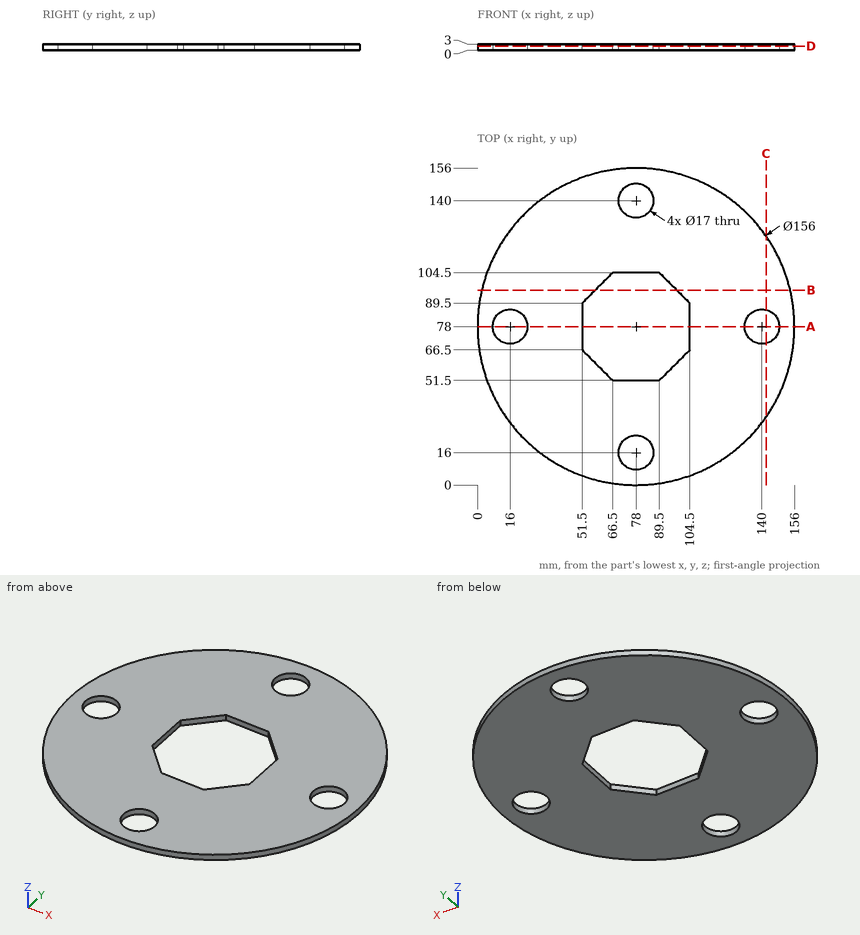
Design review of the part shown in the three views and the two pictorial views. Dimensions are in mm from the part's minimum x, y and z. Give positions to 0.01 mm unless a question says otherwise; leave off trailing zeros. Loops run counter-clockwise (first coordinate to the right, second up) from the corner with the lowest first, then second, coordinate; pieces in that order, holes last. Notation, with made-up numbers: M -2.5,27.5 L 30.5,27.5 A20 cw 30.5,65.5 Z; hole C -14.75,-35 d5. An arc over 180 degrees is marked long. Put each result on its own line as item: value. Start each with the question number.
(1) For pin 1 (0.9 mm diameter, centred on y = 81.5, z = 1.5, fed in from -X); pin 2 (1.5 mm diameter, centred on y = 72.5, z = 1, fed in from +X), all flat-tipped, find the tip position at first contact; note any pin that passes through.
(2) Wall thickness on L1, parallel to Y at x = 78, z = 1.3; L2, parallel to X at y = 79, z = 0.35; L3, parallel to Y at x = 74.5, z = 1.15: over which ranges is each line inside the solid? List them lowest first.
(3) Add section D-D, the plane z = 1.95. Write out the cut boundary in (x, y).
(4) Add section C-C, the plane x = 142. Write out the cut boundary in (y, z).
(5) Add section A-A, the plane y = 78. Write out the cut boundary in (x, z).
(6) Add section B-B, the plane y = 96. Write out the cut boundary in (x, z).
Result:
1. pin 1: stops at x = 0.06
1. pin 2: stops at x = 155.86
2. L1: y = 0 to 7.5, 24.5 to 51.5, 104.5 to 131.5, 148.5 to 156
2. L2: x = 0.01 to 7.56, 24.44 to 51.5, 104.5 to 131.56, 148.44 to 155.99
2. L3: y = 0.08 to 8.25, 23.75 to 51.5, 104.5 to 132.25, 147.75 to 155.92
3. outline: C 78,78 d156; hole C 16,78 d17; hole M 51.5,66.5 L 66.5,51.5 L 89.5,51.5 L 104.5,66.5 L 104.5,89.5 L 89.5,104.5 L 66.5,104.5 L 51.5,89.5 Z; hole C 78,16 d17; hole C 78,140 d17; hole C 140,78 d17
4. outline: M 33.41,0 L 69.74,0 L 69.74,3 L 33.41,3 Z; M 86.26,0 L 122.59,0 L 122.59,3 L 86.26,3 Z
5. outline: M 0,0 L 7.5,0 L 7.5,3 L 0,3 Z; M 24.5,0 L 51.5,0 L 51.5,3 L 24.5,3 Z; M 104.5,0 L 131.5,0 L 131.5,3 L 104.5,3 Z; M 148.5,0 L 156,0 L 156,3 L 148.5,3 Z
6. outline: M 2.11,0 L 58,0 L 58,3 L 2.11,3 Z; M 98,0 L 153.89,0 L 153.89,3 L 98,3 Z
